Model file for the job. Use its own axes, mm. A direction names the side the tool comes from. Round coordinates to 2 decimals unless told otherwise and drop trailing zeros. Order: outer loops, then holes, each group sorted by start corner. A loop starts at its lowest first (then second) coordinate and runs counter-clockwise, first axis right, second up. Notation, with made-up numbers: (10.25, 50.25) - (51.25, 50.25) arc R16 ccw to (51.25, 55.25) - close; hole circle Ø4 at (30, 65.25). An arc over 180 degrees is marked (long way). Answer as CSV lines item,"result". Start each with the question number.
1. Band-saw the part on C-C on x = -38.5. List the corners of the cut face in (y, z).
2. 3-axis set-ups, long thin cutter, end or side, ignore diameter. For faces 4 (the face through (-1, 10, -1)), 5 (the face through (-35, 3, 15)): which of +Z, -Z, +X, -X, +Y, -Y reach the whole face in a straight line?
3. Pin check, flat tips, straight feed: pin 1 Ø1.8 at (x, y) = (10, 3.5) entering from +Z; pin 2 Ø11 at (x, z) = (-10, 34.5) entering from -Y; pin 3 Ø11 at (x, z) = (-35.5, 28.5) entering from -Y. Stop position of each tip, or through.
4. Band-saw the part on B-B on y = 1.5. List the corners of the cut face in (x, z) (3 decimals).
5. Band-saw the part on A-A on z = 31. List the corners of the cut face in (x, y) (3 decimals), then the cut area to 3 significant figures.
6. Wall check: line 1 along X through (y, z) = (2, 41.5) (3 decimals); line 2 along Z through (x, y) = (-10, 5.5); line 3 along Y through (x, z) = (-28.5, 37.5). Give the ranges that are in metal, low to high. Write a range as [from, to].
7. Pull direction X, two halves, no side cores. Call faces 1 (the face through (41.995, 3, 33)), 2 (the face through (-52.5, 5, 1)), 3 (the face through (-1, 5, -50)): released by +X, released by -X, zero draft, split by the parting line, or undercut.
```python
from build123d import *

# Parameters (mm, degrees)
SKETCH1_W           = 105
SKETCH1_H           = 100
BOSS_EXTRUDE1_DEPTH = 10
SKETCH2_W           = 14
SKETCH2_H           = 6
CUT_EXTRUDE1_DEPTH  = 35


with BuildPart() as part:
    # Sketch1 → Boss-Extrude1 (new body)
    with BuildSketch(Plane(origin=(0, 0, 0), x_dir=(1, 0, 0), z_dir=(0, 1, 0))):
        Rectangle(SKETCH1_W, SKETCH1_H)
    extrude(amount=BOSS_EXTRUDE1_DEPTH)

    # Sketch2 → Cut-Extrude1 (cut)
    with BuildSketch(Plane.XY.offset(50)):
        with Locations((-34.995, 3)):
            Rectangle(SKETCH2_W, SKETCH2_H)
        with Locations((-11.665, 3)):
            Rectangle(SKETCH2_W, SKETCH2_H)
        with Locations((34.995, 3)):
            Rectangle(SKETCH2_W, SKETCH2_H)
        with Locations((11.665, 3)):
            Rectangle(SKETCH2_W, SKETCH2_H)
    extrude(amount=-CUT_EXTRUDE1_DEPTH, mode=Mode.SUBTRACT)


solid = part.part
```
Reply:
1,outline,"(0, -50) - (10, -50) - (10, 50) - (6, 50) - (6, 15) - (0, 15) - close"
2,face 4,"+Z, -Z, +X, -X, +Y"
2,face 5,"+Z, -Y"
3,pin 1,"stops at z = 15"
3,pin 2,"stops at y = 0"
3,pin 3,"stops at y = 6"
4,outline,"(-52.5, -50) - (52.5, -50) - (52.5, 50) - (41.995, 50) - (41.995, 15) - (27.995, 15) - (27.995, 50) - (18.665, 50) - (18.665, 15) - (4.665, 15) - (4.665, 50) - (-4.665, 50) - (-4.665, 15) - (-18.665, 15) - (-18.665, 50) - (-27.995, 50) - (-27.995, 15) - (-41.995, 15) - (-41.995, 50) - (-52.5, 50) - close"
5,outline,"(-52.5, 0) - (-41.995, 0) - (-41.995, 6) - (-27.995, 6) - (-27.995, 0) - (-18.665, 0) - (-18.665, 6) - (-4.665, 6) - (-4.665, 0) - (4.665, 0) - (4.665, 6) - (18.665, 6) - (18.665, 0) - (27.995, 0) - (27.995, 6) - (41.995, 6) - (41.995, 0) - (52.5, 0) - (52.5, 10) - (-52.5, 10) - close"
5,area,"714 mm2"
6,line 1,"x = [-52.5, -41.995], [-27.995, -18.665], [-4.665, 4.665], [18.665, 27.995], [41.995, 52.5]"
6,line 2,"z = [-50, 15]"
6,line 3,"y = [6, 10]"
7,face 1,"undercut"
7,face 2,"released by -X"
7,face 3,"zero draft"
